Geometry: final body of the model. Coordinates: model frame, mm. Face numbers are marked on the shaded views. A direction names the side the tool comes from. Round coordinates to 2 decimals unless told otherwise and drop trailing zeros. Loops run counter-clockwise (first coordinate to the right, second up) from the corner with the lowest first, then second, coordinate; pieces in that order, holes last. Notation, with made-up numbers: (86.25, 51) - (118.25, 51) arc R29 ccw to (118.25, 76) - close; hole circle Ø11 at (59, 15.5). An arc over 180 degrees is marked (long way). Answer as CSV lines item,"result".
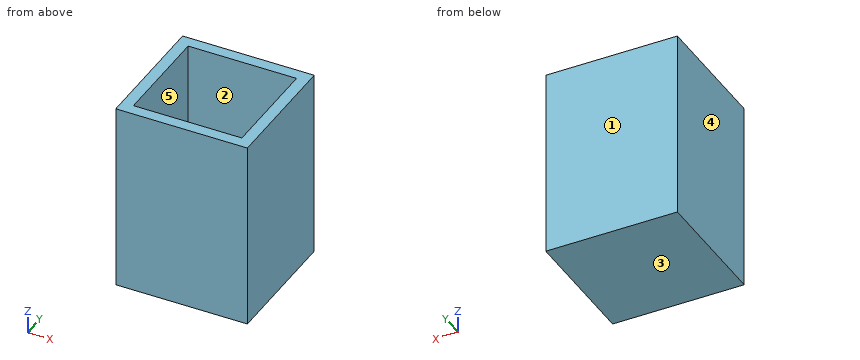
Autodesk Fusion 360 part; units mm, degrees
sketch "Sketch1" plane through (0, 0, 0) normal (0, 0, 1) x (1, 0, 0)
  line L0 (0, 0) -> (34, 0)
  line L1 (34, 0) -> (34, 33)
  line L2 (34, 33) -> (0, 33)
  line L3 (0, 33) -> (0, 0)
  dimension "d1" = 33
  dimension "d2" = 34
extrude "Extrude1" add sketch "Sketch1" along normal blind 49
shell "Shell1" thickness 3 removed faces 1 at (11.3333, 22, 49)
(1) Draft query along Y for the marked faces 1, 2 and 3. Return one class per face: pulls with the +Y half, pulls with the -Y half, needs draft (parallel to the pull), parting line crosses it, or undercut.
Findings below:
face 1,"pulls with the +Y half"
face 2,"undercut"
face 3,"needs draft"
(2) Material intervals for line 1 along Y through (x, z) = (14.5, 47); line 2 along X through (y, z) = (19, 41); line 3 along Z through (x, y) = (4, 18.5), sorted ascending.
Findings below:
line 1,"0 to 3, 30 to 33"
line 2,"0 to 3, 31 to 34"
line 3,"0 to 3"
(3) Section B-B (z = 25.5). Output: boundary loops of the cut face in (x, y), and give its area (3 significant figures).
Findings below:
outline,"(0, 0) - (34, 0) - (34, 33) - (0, 33) - close; hole (3, 3) - (31, 3) - (31, 30) - (3, 30) - close"
area,"366 mm2"
(4) Section C-C (x = 10). Output: boundary loops of the cut face in (y, z).
Findings below:
outline,"(0, 0) - (33, 0) - (33, 49) - (30, 49) - (30, 3) - (3, 3) - (3, 49) - (0, 49) - close"
(5) Section A-A (y = 20). Output: boundary loops of the cut face in (x, z), and give its area (3 significant figures).
Findings below:
outline,"(0, 0) - (34, 0) - (34, 49) - (31, 49) - (31, 3) - (3, 3) - (3, 49) - (0, 49) - close"
area,"378 mm2"
(6) Pin query (flat end, axial travel): P1, Ø4, axis at x = 27.5, y = 10.5, coming from the +Z side. Return the tip coordinate at first contact, or that it passes through.
Findings below:
P1,"z = 3"
(7) Access query for the marked faces 4 and 5. Directions: +Z, -Z, +X, -X, +Y, -Y. A direction counts if a zero-diameter tool reaches every point of the face in a straight line with its end or side. Return the directions, or none.
Findings below:
face 4,"+Z, -Z, -X, +Y, -Y"
face 5,"+Z"
